from build123d import *

# Parameters (mm, degrees)
F0_W     = 11.5
F0_H     = 14
F0_W_2   = 7
F0_H_2   = 5
F1_DEPTH = 7
F2_R     = 1


with BuildPart() as f1:
    # F0 (on Top) → F1 (new body)
    with BuildSketch(Plane.XY):
        with Locations((0, 0.5)):
            Rectangle(F0_W, F0_H)
        Rectangle(F0_W_2, F0_H_2, mode=Mode.SUBTRACT)
    extrude(amount=F1_DEPTH)

    # F2
    f2_edges = [f1.edges().sort_by_distance(p)[0] for p in [
        (-5.75, -6.5, 3.5),
        (5.75, -6.5, 3.5),
        (5.75, 7.5, 3.5),
        (-5.75, 7.5, 3.5),
    ]]
    fillet(f2_edges, radius=F2_R)


solid = f1.part
Check sheet for the modelled part. Datum: model origin and axes. Units: mm. A direction names the side the tool comes from. Coordinates: 2 decimals unless noted, no trailing zeros. Loops run counter-clockwise (first coordinate to the right, second up) from the corner with the lowest first, then second, coordinate; pieces in that order, holes last. Notation, with made-up numbers: (43, 19.25) -> (68, 19.25) arc R26 cw to (68, 36.25) -> close; hole circle Ø4 at (47.25, -34.75). An arc over 180 degrees is marked (long way). Write item = value, one per line. Start each with the question number.
1. Section check A-A on x = 3.25. Record the cut outline in (y, z).
2. Draft check along X on faces 3 (the cylindrical face through (-5.465, 7.199, 3.549)), 4 (the flat face through (0, 7.5, 3)), 5 (the cylindrical face through (5.449, -6.215, 3.549)), 6 (the flat face through (-3.5, 0, 3)). Enter one of: released by +X, released by -X, zero draft, split by the parting line, or undercut.
3. Material ranges on line 1 (Y direction, x = -3.25, z = 2.5); line 2 (X direction, y = 0, z = 1); line 3 (Y direction, x = -5, z = 2.25), recorded low to high.
4. Section check C-C on y = 1. Record the cut outline in (x, z), then the cut area to 3 significant figures.
5. Section check B-B on z = 4. Record the cut outline in (x, y).
6. Tool access check on faces 1 (the flat face through (3.5, 0, 3)), 2 (the flat face through (0, 4, 0)). Record the directions out of +Z, -Z, +X, -X, +Y, -Y that give a thin tool (end or side, any length) a straight path to the whole face; none if there is none.
Responses:
q1.outline = (-6.5, 0) -> (-2.5, 0) -> (-2.5, 7) -> (-6.5, 7) -> close; (2.5, 0) -> (7.5, 0) -> (7.5, 7) -> (2.5, 7) -> close
q2.face_3 = released by -X
q2.face_4 = zero draft
q2.face_5 = released by +X
q2.face_6 = undercut
q3.line_1 = -6.5 to -2.5, 2.5 to 7.5
q3.line_2 = -5.75 to -3.5, 3.5 to 5.75
q3.line_3 = -6.47 to 7.47
q4.outline = (-5.75, 0) -> (-3.5, 0) -> (-3.5, 7) -> (-5.75, 7) -> close; (3.5, 0) -> (5.75, 0) -> (5.75, 7) -> (3.5, 7) -> close
q4.area = 31.5 mm2
q5.outline = (-5.75, -5.5) arc R1 ccw to (-4.75, -6.5) -> (4.75, -6.5) arc R1 ccw to (5.75, -5.5) -> (5.75, 6.5) arc R1 ccw to (4.75, 7.5) -> (-4.75, 7.5) arc R1 ccw to (-5.75, 6.5) -> close; hole (-3.5, -2.5) -> (3.5, -2.5) -> (3.5, 2.5) -> (-3.5, 2.5) -> close
q6.face_1 = +Z, -Z
q6.face_2 = -Z, +X, -X, +Y, -Y
